Build history of the part. All positions in model axes, mm. A direction names the side the tool comes from. Give positions to 0.01 mm unless a question says otherwise; leave off trailing zeros. Order: outer loops, then holes, each group sorted by start corner. A loop starts at its lowest first (then second) coordinate and runs counter-clockwise, first axis right, second up. Notation, with made-up numbers: (57, 35) - (81, 35) arc R16 cw to (81, 50) - close; hole circle Ø5 at (-16, 41.25). An arc over 180 degrees is marked (long way). Write each question's results on one line, items separated by ' | '. Start each with the question number.
1) Drill centre line: line 1 along X through (y, z) = (33, 0.75). Where is it in solid material? Low to high. Write a range as from..to.
2) Cut at D-D on x = -7.5. State how many separate pieces and enclosed holes the cut face has, plus the area to 3 significant figures.
3) Cut at C-C on z = 0. List the corners of the cut face in (x, y).
4) Cut at A-A on x = 2.25. List the corners of the cut face in (y, z), plus the area to 3 significant figures.
5) Cut at B-B on y = 37.5. List the corners of the cut face in (x, z).
6) Tool access for faces 4 (the face through (11, -1, 0)), 5 (the face through (-11.74, -34.452, 7.934)): list every direction of +Z, -Z, +X, -X, +Y, -Y with a clear straight run to the whole face (end or side of a thin tool).
7) Two-plate mould, pull along Y, no slides. Class faces 1 (the face through (-11.74, -44.452, -7.066)), 2 (the face through (-12.5, -1, 0)), 3 (the face through (-11.2, 47.5, -0.1)): +Y half, -Y half, draft (parallel to the pull), parting line (faces both ways), or undercut.
8) Drop a flat-ended pin along its axis: pin 1 Ø6.5 at (y, z) = (-22.5, -7.5) entering from +X. Give the stop position or say it passes through.
from build123d import *

# Parameters (mm, degrees)
BOSS_EXTRUDE1_DEPTH      = 47.5
BOSS_EXTRUDE1_DEPTH_BACK = 47.5
SKETCH3_W                = 25
SKETCH3_H                = 25
SKETCH3_W_2              = 22
SKETCH3_H_2              = 22
SKETCH6_R                = 2
CUT_EXTRUDE3_DEPTH       = 25
SKETCH7_R                = 2
CUT_EXTRUDE4_DEPTH       = 25
SKETCH8_R                = 2
CUT_EXTRUDE5_DEPTH       = 25


with BuildPart() as part:
    # Sketch3 → Boss-Extrude1 (new, two sides: drawn at the far end of the back side and taken through both)
    with BuildSketch(Plane(origin=(0, 0, 0), x_dir=(1, 0, 0), z_dir=(0, 1, 0)).offset(-BOSS_EXTRUDE1_DEPTH_BACK)):
        Rectangle(SKETCH3_W, SKETCH3_H)
        Rectangle(SKETCH3_W_2, SKETCH3_H_2, mode=Mode.SUBTRACT)
    extrude(amount=BOSS_EXTRUDE1_DEPTH + BOSS_EXTRUDE1_DEPTH_BACK)

    # Sketch6 → Cut-Extrude3 (cut)
    with BuildSketch(Plane(origin=(12.5, 0, 0), x_dir=(0, 0, -1), z_dir=(1, 0, 0))):
        with Locations((7.5, -42.5)):
            Circle(SKETCH6_R)
        with Locations((7.5, -22.5)):
            Circle(SKETCH6_R)
        with Locations((-7.5, -42.5)):
            Circle(SKETCH6_R)
        with Locations((-7.5, -22.5)):
            Circle(SKETCH6_R)
        with Locations((7.5, -32.5)):
            Circle(SKETCH6_R)
        with Locations((-7.5, -32.5)):
            Circle(SKETCH6_R)
    extrude(amount=-CUT_EXTRUDE3_DEPTH, mode=Mode.SUBTRACT)

    # Sketch7 → Cut-Extrude4 (cut)
    with BuildSketch(Plane(origin=(0, 0, -12.5), x_dir=(-1, 0, 0), z_dir=(0, 0, -1))):
        with Locations((7.5, 37.5)):
            Circle(SKETCH7_R)
        with Locations((7.5, 27.5)):
            Circle(SKETCH7_R)
        with Locations((-7.5, 37.5)):
            Circle(SKETCH7_R)
        with Locations((-7.5, 27.5)):
            Circle(SKETCH7_R)
        with Locations((-7.5, 17.5)):
            Circle(SKETCH7_R)
        with Locations((7.5, 17.5)):
            Circle(SKETCH7_R)
    extrude(amount=-CUT_EXTRUDE4_DEPTH, mode=Mode.SUBTRACT)

    # Sketch8 → Cut-Extrude5 (cut)
    with BuildSketch(Plane(origin=(12.5, 0, 0), x_dir=(0, 0, -1), z_dir=(1, 0, 0))):
        with Locations((5.5, 40.5)):
            Circle(SKETCH8_R)
        with Locations((5.5, 29.5)):
            Circle(SKETCH8_R)
        with Locations((-5.5, 29.5)):
            Circle(SKETCH8_R)
        with Locations((-5.5, 40.5)):
            Circle(SKETCH8_R)
    extrude(amount=-CUT_EXTRUDE5_DEPTH, mode=Mode.SUBTRACT)


solid = part.part
Results:
1) line 1: -12.5..-11, 11..12.5
2) separate pieces: 8 | enclosed holes: 0 | area: 249 mm^2
3) outline: (-12.5, -47.5) - (-11, -47.5) - (-11, 47.5) - (-12.5, 47.5) - close; (11, -47.5) - (12.5, -47.5) - (12.5, 47.5) - (11, 47.5) - close
4) outline: (-47.5, -12.5) - (47.5, -12.5) - (47.5, -11) - (-47.5, -11) - close; (-47.5, 11) - (47.5, 11) - (47.5, 12.5) - (-47.5, 12.5) - close | area: 285 mm^2
5) outline: (-12.5, -12.5) - (-9.5, -12.5) - (-9.5, -11) - (-11, -11) - (-11, 11) - (-9.5, 11) - (-9.5, 12.5) - (-12.5, 12.5) - close; (-5.5, -12.5) - (5.5, -12.5) - (5.5, -11) - (-5.5, -11) - close; (-5.5, 11) - (5.5, 11) - (5.5, 12.5) - (-5.5, 12.5) - close; (9.5, -12.5) - (12.5, -12.5) - (12.5, 12.5) - (9.5, 12.5) - (9.5, 11) - (11, 11) - (11, -11) - (9.5, -11) - close
6) face 4: +Y, -Y | face 5: +X, -X
7) face 1: undercut | face 2: draft | face 3: +Y half
8) pin 1: x = 12.5
